from build123d import *

# Parameters (mm, degrees)
RESSALTO_EXTRUS_O1_DEPTH = 2
ESBO_O2_W                = 15
ESBO_O2_H                = 0.4
CORTE_EXTRUS_O1_DEPTH    = 0.1
PADR_O_LINEAR1_COUNT     = 6
PADR_O_LINEAR1_PITCH     = 4


with BuildPart() as part:
    # Esboço1 → Ressalto-extrusão1 (new body)
    with BuildSketch(Plane(origin=(0, 0, 0), x_dir=(1, 0, 0), z_dir=(0, 1, 0))):
        with BuildLine():
            Line((1.674494665, 0), (28.325505335, 0))
            ThreePointArc((28.325505335, 0), (29.609412934, -0.466513359), (30.294360486, -1.648418723))
            Line((30.294360486, -1.648418723), (34.580074772, -25.648418723))
            ThreePointArc((34.580074772, -25.648418723), (34.144706262, -27.283907599), (32.611219621, -28))
            ThreePointArc((32.611219621, -28), (15.082885827, -27.269989968), (-2.446011347, -27.98634468))
            ThreePointArc((-2.446011347, -27.98634468), (-4.089503342, -27.338819548), (-4.578838652, -25.641496454))
            Line((-4.578838652, -25.641496454), (-0.294360486, -1.648418723))
            ThreePointArc((-0.294360486, -1.648418723), (0.390587066, -0.466513359), (1.674494665, 0))
        make_face()
        with BuildLine():
            Line((5, -5.5), (5, -19.5))
            ThreePointArc((5, -19.5), (4, -20.5), (3, -19.5))
            Line((3, -19.5), (3, -5.5))
            ThreePointArc((3, -5.5), (4, -4.5), (5, -5.5))
        make_face(mode=Mode.SUBTRACT)
        with BuildLine():
            Line((25, -5.5), (25, -19.5))
            ThreePointArc((25, -19.5), (26, -20.5), (27, -19.5))
            Line((27, -19.5), (27, -5.5))
            ThreePointArc((27, -5.5), (26, -4.5), (25, -5.5))
        make_face(mode=Mode.SUBTRACT)
    extrude(amount=RESSALTO_EXTRUS_O1_DEPTH)

    # Esboço2 → Corte-extrusão1 (cut)
    with BuildSketch(Plane(origin=(0, 2, 0), x_dir=(1, 0, 0), z_dir=(0, 1, 0))):
        with Locations((15, -23.969622092)):
            Rectangle(ESBO_O2_W, ESBO_O2_H)
    corte_extrus_o1 = extrude(amount=-CORTE_EXTRUS_O1_DEPTH, mode=Mode.SUBTRACT)

    # Padrão linear1: Corte-extrusão1 ×6
    with Locations(*[(0, 0, -i * PADR_O_LINEAR1_PITCH) for i in range(1, PADR_O_LINEAR1_COUNT)]):
        add(corte_extrus_o1, mode=Mode.SUBTRACT)


solid = part.part
Input: part model. Units: mm. Frame: model coordinates. A direction names the side the tool comes from. Round coordinates to 2 decimals unless told otherwise and drop trailing zeros. Loops run counter-clockwise (first coordinate to the right, second up) from the corner with the lowest first, then second, coordinate; pieces in that order, holes last. Notation, with made-up numbers: (66.25, -9) -> (85.25, -9) arc R34 ccw to (85.25, 30) -> close; hole circle Ø10 at (45.5, 84). An arc over 180 degrees is marked (long way). Answer as a JSON object with one key per item and string values. Group by question number.
1) Pin query (flat end, axial travel): pin 1 (2 mm diameter, centred on x = 17, z = 7.5, fed in from -Y); pin 2 (1 mm diameter, centred on y = 1.5, z = 21.5, fed in from +X); pin 3 (0.6 mm diameter, centred on y = 1, z = 9.5, fed in from -X). Return the tip coordinate at first contact, or that it passes through.
2) Draft query along X for faces 1 (the flat face through (5, 1, 12)), 2 (the cylindrical face through (15.33, 0.99, 27.27)), 3 (the flat face through (32.407, 0.986, 13.48)), 4 (the flat face through (15, 2, 14)). Return one class per face: +X half, -X half, draft (parallel to the pull), parting line (faces both ways), or undercut.
3) Section query A-A on x = 4. Output: boundary loops of the cut face in (y, z).
4) Section query B-B on z = 9.25. Output: boundary loops of the cut face in (x, y), plus the area to 3 significant figures.
5) Ray query, L1, parallel to X at y = 0.3, z = 5; L2, parallel to X at y = 1.6, z = 16.75; L3, parallel to Z at x = 30, y = 0.2. Return the intervals inside material, ascending.
6) Reachability of faces 5 (the cylindrical face through (0.376, 0.986, 0.479)), 6 (the cylindrical face through (4, 1, 4.5)) from +Z, -Z, +X, -X, +Y, -Y: full face, straight path, thin tool, end or side. Return the list, or none.
7) Section query D-D on x = 10.5. Output: boundary loops of the cut face in (y, z).
8) Section query C-C on y = 1.15. Output: boundary loops of the cut face in (x, z).
Reply:
{
 "1": {"pin 1": "stops at y = 0", "pin 2": "stops at x = 33.93", "pin 3": "stops at x = -1.75"},
 "2": {"face 1": "undercut", "face 2": "undercut", "face 3": "+X half", "face 4": "draft"},
 "3": {"outline": "(0, 0) -> (2, 0) -> (2, 4.5) -> (0, 4.5) -> close; (0, 20.5) -> (2, 20.5) -> (2, 27.55) -> (0, 27.55) -> close"},
 "4": {"outline": "(-1.65, 0) -> (3, 0) -> (3, 2) -> (-1.65, 2) -> close; (5, 0) -> (25, 0) -> (25, 2) -> (5, 2) -> close; (27, 0) -> (31.65, 0) -> (31.65, 2) -> (27, 2) -> close", "area": "58.6 mm2"},
 "5": {"L1": "x = -0.89 to 3.13, 4.87 to 25.13, 26.87 to 30.89", "L2": "x = -2.99 to 3, 5 to 25, 27 to 32.99", "L3": "z = 0.91 to 27.8"},
 "6": {"face 5": "-Z, -X, +Y, -Y", "face 6": "+Y, -Y"},
 "7": {"outline": "(0, 0) -> (2, 0) -> (2, 3.77) -> (1.9, 3.77) -> (1.9, 4.17) -> (2, 4.17) -> (2, 7.77) -> (1.9, 7.77) -> (1.9, 8.17) -> (2, 8.17) -> (2, 11.77) -> (1.9, 11.77) -> (1.9, 12.17) -> (2, 12.17) -> (2, 15.77) -> (1.9, 15.77) -> (1.9, 16.17) -> (2, 16.17) -> (2, 19.77) -> (1.9, 19.77) -> (1.9, 20.17) -> (2, 20.17) -> (2, 23.77) -> (1.9, 23.77) -> (1.9, 24.17) -> (2, 24.17) -> (2, 27.32) -> (0, 27.32) -> close"},
 "8": {"outline": "(-4.58, 25.64) -> (-0.29, 1.65) arc R2 ccw to (1.67, 0) -> (28.33, 0) arc R2 ccw to (30.29, 1.65) -> (34.58, 25.65) arc R2 ccw to (32.61, 28) arc R212.79 cw to (-2.45, 27.99) arc R2 ccw to start; hole (3, 5.5) arc R1 ccw to (5, 5.5) -> (5, 19.5) arc R1 ccw to (3, 19.5) -> close; hole (25, 5.5) arc R1 ccw to (27, 5.5) -> (27, 19.5) arc R1 ccw to (25, 19.5) -> close"}
}
